```python
from build123d import *

# Parameters (mm, degrees)
ESBO_O4_W                = 11.8
ESBO_O4_H                = 4
RESSALTO_EXTRUS_O2_DEPTH = 5.26
ESBO_O5_R                = 2
RESSALTO_EXTRUS_O4_DEPTH = 6.74


with BuildPart() as part:
    # Esboço4 → Ressalto-extrusão2 (new body)
    with BuildSketch(Plane.XY.offset(6.74)):
        with Locations((70.144771166, -37.321923077)):
            Rectangle(ESBO_O4_W, ESBO_O4_H)
    extrude(amount=RESSALTO_EXTRUS_O2_DEPTH)

    # Esboço5 → Ressalto-extrusão4 (add)
    with BuildSketch(Plane(origin=(0, 0, 6.74), x_dir=(-1, 0, 0), z_dir=(0, 0, -1))):
        with Locations(Location((-70.144771166, -37.321923077, 0), (0, 0, 270))):
            Circle(ESBO_O5_R)
    extrude(amount=RESSALTO_EXTRUS_O4_DEPTH)


solid = part.part
```
Can you work these out from the model? Positions are in its coordinate system, mm. A direction names the side the tool comes from. Round coordinates to 2 decimals unless told otherwise and drop trailing zeros. Order: outer loops, then holes, each group sorted by start corner. A loop starts at its lowest first (then second) coordinate and runs counter-clockwise, first axis right, second up.
(1) If we section it at A-A (x = 69.5): Please give me the cut outline in (y, z).
Results are:
outline: (-39.32, 6.74) - (-39.22, 6.74) - (-39.22, 0) - (-35.43, 0) - (-35.43, 6.74) - (-35.32, 6.74) - (-35.32, 12) - (-39.32, 12) - close
(2) I'm going to push flat-ended pins straight in: pin 1 (1.5 mm diameter, centred on y = -36.5, z = 5, fed in from -X); pin 2 (1 mm diameter, centred on y = -39, z = 4, fed in from -X). Where does each tip first touch, or does it pass through?
Results are:
pin 1: stops at x = 68.15
pin 2: stops at x = 68.53
(3) If we section it at C-C (z = 3.5): Please give me the cut outline in (x, y).
Results are:
outline: circle Ø4 at (70.14, -37.32)
(4) If we section it at D-D (x = 67): Please give me the cut outline in (y, z).
Results are:
outline: (-39.32, 6.74) - (-35.32, 6.74) - (-35.32, 12) - (-39.32, 12) - close
(5) If we section it at B-B (y = -35.9): Please give me the cut outline in (x, z), plus the area to 3 significant figures.
Results are:
outline: (64.24, 6.74) - (68.74, 6.74) - (68.74, 0) - (71.55, 0) - (71.55, 6.74) - (76.04, 6.74) - (76.04, 12) - (64.24, 12) - close
area: 81.0 mm2
(6) If I drill on L1, parallel to Z at x = 66, y = -39; L2, parallel to Y at x = 70.25, z = 4; L3, parallel to X at y = -37.3, z = 1.5, over which ranges is the centre line in solid material (lowest first)?
Results are:
L1: z = 6.74 to 12
L2: y = -39.32 to -35.32
L3: x = 68.14 to 72.14
(7) On a 3-axis mill with a long thin cutter (end or side, diameter ignored), from which of +Z, -Z, +X, -X, +Y, -Y can I reach the whole of each face in a straight line? I mean faces 1 (the face through (68.46, -38.4, 3.42)), 2 (the face through (76.045, -37, 9)). Say none if no direction works.
Results are:
face 1: -Z
face 2: +Z, -Z, +X, +Y, -Y
